Source: CAD feature listing. Evaluate the final solid. Frame: model axes, mm. Round coordinates to 2 decimals unless told otherwise and drop trailing zeros. Write each loop counter-clockwise with the first axis right and the second up, starting at its lowest first coordinate (ties: lowest second). Pieces come first, ordered by that corner, then holes. Notation, with made-up numbers: (-23.5, -32.5) - (-13.5, -32.5) arc R19 ccw to (-13.5, -21.5) - close; hole circle Ø11 at (41.5, -24.75). An arc over 180 degrees is marked (long way). Write item = value, one per line. Start each with the question number.
```python
from build123d import *

# Parameters (mm, degrees)
F1_DEPTH = 3.175
F2_W     = 3.175
F2_H     = 114.3
F3_DEPTH = 3.175
F4_W     = 76.2
F4_H     = 161.842626
F5_DEPTH = 3.176


with BuildPart() as f1:
    # F0 (on Front) → F1 (new body)
    with BuildSketch(Plane.XZ):
        Polygon((228.6, -304.8), (276.225, -304.8), (276.225, 190.5), (279.4, 190.5), (279.4, 266.7), (276.225, 266.7), (-276.225, 266.7), (-279.4, 266.7), (-279.4, 190.5), (-276.225, 190.5), (-276.225, 185.04481), (-276.225, -304.8), (-228.6, -304.8), (-228.6, -38.1), (-152.4, -38.1), (-152.4, -304.8), (152.4, -304.8), (152.4, -38.1), (228.6, -38.1), align=None)
    extrude(amount=F1_DEPTH)

    # F2 (on face) → F3 (join, through all)
    with BuildSketch(Plane.XZ.offset(3.175)):
        with Locations((280.9875, 209.55)):
            Rectangle(F2_W, F2_H)
        with Locations((-280.9875, 209.55)):
            Rectangle(F2_W, F2_H)
    extrude(amount=-F3_DEPTH)

    # F4 (on face) → F5 (cut, through all)
    with BuildSketch(Plane.XZ.offset(3.175)):
        Polygon((-228.6, -142.957374), (-228.6, -38.1), (-237.773832, -142.957374), (-267.051168, -142.957374), (-276.225, -38.1), (-276.225, -142.957374), (-276.225, -304.8), (-252.891773, -304.8), (-251.933227, -304.8), (-228.6, -304.8), align=None)
        with Locations((-190.5, -223.878687)):
            Rectangle(F4_W, F4_H)
        Polygon((-152.4, -38.1), (-152.4, -142.957374), (-152.4, -304.8), (152.4, -304.8), (152.4, -142.957374), (152.4, -38.1), (145.741312, -114.209149), (143.226168, -142.957374), (-143.226168, -142.957374), (-145.741312, -114.209149), align=None)
        with Locations((190.5, -223.878687)):
            Rectangle(F4_W, F4_H)
        Polygon((228.6, -142.957374), (228.6, -304.8), (251.933227, -304.8), (252.891773, -304.8), (276.225, -304.8), (276.225, -142.957374), (276.225, -38.1), (267.051168, -142.957374), (237.773832, -142.957374), (228.6, -38.1), align=None)
    extrude(amount=-F5_DEPTH, mode=Mode.SUBTRACT)


solid = f1.part
```
(1) Ray query, L1, parallel to X at y = -0.8, z = 169 (3 decimals); L2, parallel to X at y = -0.7, z = -92; L3, parallel to Z at x = -220, y = -1.8. Return the intervals inside material, ascending. Write a range as from..to.
(2) Section A-A (z = -56). Return the cut outline in (x, y) (3 decimals).
(3) Section C-C (x = -161.5). Return the cut outline in (y, z) (3 decimals).
(4) Section B-B (y = -2.55). Return the cut outline in (x, z) (3 decimals).
(5) Contact query for flat-ended pins moving along their axis: P1, Ø1, axis at x = 178, y = -2, coming from the -Z side; P2, Ø1, axis at x = 278, y = -1, coming from the -Z side; P3, Ø1.6, axis at y = -1, z = 103, coming from the +X side (3 decimals). Output: stop coordinate, or through.
(6) Section D-D (z = 66). Return the cut outline in (x, y) (3 decimals).
Solution:
q1.L1 = -282.575..-279.4, -276.225..276.225, 279.4..282.575
q1.L2 = -271.51..-233.32, -147.68..147.68, 233.32..271.51
q1.L3 = -38.1..266.7
q2.outline = (-274.659, -3.175) - (-230.166, -3.175) - (-230.166, 0) - (-274.659, 0) - close; (-150.834, -3.175) - (150.834, -3.175) - (150.834, 0) - (-150.834, 0) - close; (230.166, -3.175) - (274.659, -3.175) - (274.659, 0) - (230.166, 0) - close
q3.outline = (-3.175, -38.1) - (0, -38.1) - (0, 266.7) - (-3.175, 266.7) - close
q4.outline = (-282.575, 152.4) - (-279.4, 152.4) - (-279.4, 190.5) - (-276.225, 190.5) - (-276.225, -38.1) - (-267.051, -142.957) - (-237.774, -142.957) - (-228.6, -38.1) - (-152.4, -38.1) - (-143.226, -142.957) - (143.226, -142.957) - (152.4, -38.1) - (228.6, -38.1) - (237.774, -142.957) - (267.051, -142.957) - (276.225, -38.1) - (276.225, 190.5) - (279.4, 190.5) - (279.4, 152.4) - (282.575, 152.4) - (282.575, 266.7) - (-282.575, 266.7) - close
q5.P1 = -38.1
q5.P2 = 190.5
q5.P3 = 276.225
q6.outline = (-276.225, -3.175) - (276.225, -3.175) - (276.225, 0) - (-276.225, 0) - close
